```python
from build123d import *

# Parameters (mm, degrees)
REVOLVE_1_ANGLE          = 180
CUT_EXTRUDE_3_DEPTH      = 14.509996299
CUT_EXTRUDE_3_DEPTH_BACK = 14.509996299
SKETCH_5_W               = 6
SKETCH_5_H               = 20
SKETCH_11_R              = 5.65
CUT_EXTRUDE_7_DEPTH      = 13.325988804
SKETCH_12_R              = 6.25
CUT_EXTRUDE_8_DEPTH      = 2


with BuildPart() as part:
    # 草图1 → 旋转1 (revolve)
    with BuildSketch(Plane(origin=(0, 0, 0), x_dir=(0, 0, -1), z_dir=(1, 0, 0))):
        with BuildLine():
            Line((0, 7.8), (0, -7.8))
            ThreePointArc((0, -7.8), (-7.8, 0), (0, 7.8))
        make_face()
    revolve(axis=Axis((0, 7.8, 0), (0, -1, 0)), revolution_arc=REVOLVE_1_ANGLE)

    # 草图5 → 切除-拉伸3 (cut, two sides: drawn at the far end of the back side and taken through both)
    with BuildSketch(Plane.XY.offset(-CUT_EXTRUDE_3_DEPTH_BACK)):
        with Locations((-8.5, 0.096965289)):
            Rectangle(SKETCH_5_W, SKETCH_5_H)
    extrude(amount=CUT_EXTRUDE_3_DEPTH + CUT_EXTRUDE_3_DEPTH_BACK, mode=Mode.SUBTRACT)

    # 草图11 → 切除-拉伸7 (cut, through all)
    with BuildSketch(Plane(origin=(0, 0, 0), x_dir=(0, 0, -1), z_dir=(1, 0, 0))):
        Circle(SKETCH_11_R)
    extrude(amount=-CUT_EXTRUDE_7_DEPTH, mode=Mode.SUBTRACT)

    # 草图12 → 切除-拉伸8 (cut)
    with BuildSketch(Plane(origin=(0, 0, 0), x_dir=(0, 0, -1), z_dir=(1, 0, 0))):
        Circle(SKETCH_12_R)
    extrude(amount=-CUT_EXTRUDE_8_DEPTH, mode=Mode.SUBTRACT)


solid = part.part
```
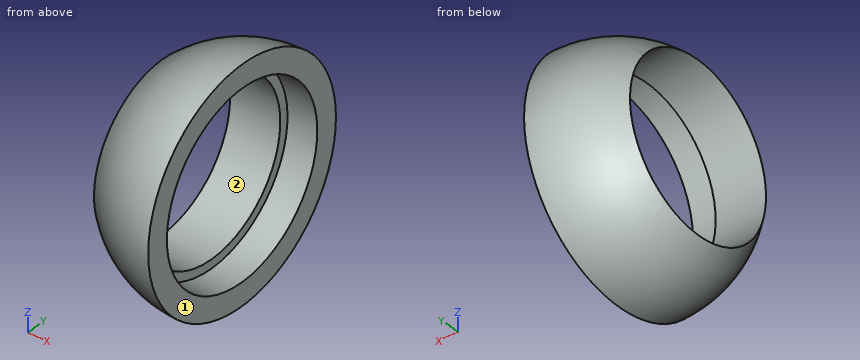
Input: part model. Units: mm. Frame: model coordinates. Face numbers are marked on the shaded views. Round coordinates to 2 decimals unless told otherwise and drop trailing zeros. Loops run counter-clockwise (first coordinate to the right, second up) from the corner with the lowest first, then second, coordinate; pieces in that order, holes last. Notation, with made-up numbers: (-12, -31.5) -> (7, -31.5) arc R31 cw to (7, -0.5) -> close; hole circle Ø11 at (84, -6.5). An arc over 180 degrees is marked (long way). One line per item, written item: value.
(1) Section D-D (z = 6.5). Return the cut outline in (x, y).
Geometry check:
outline: (0, -4.31) -> (0, 4.31) arc R4.31 ccw to start
(2) Pin query (flat end, axial travel): pin 1 (1.5 mm diameter, centred on x = -4, z = -5, fed in from -Y); pin 2 (6 mm diameter, centred on y = 2, z = 0, fed in from +X). Return the tip coordinate at first contact, or that it passes through.
Geometry check:
pin 1: y = -5.37
pin 2: through
(3) Section A-A (z = 0). Return the cut outline in (x, y), plus the area to 3 significant figures.
Geometry check:
outline: (-5.38, -5.65) arc R7.8 ccw to (0, -7.8) -> (0, -6.25) -> (-2, -6.25) -> (-2, -5.65) -> close; (-5.38, 5.65) -> (-2, 5.65) -> (-2, 6.25) -> (0, 6.25) -> (0, 7.8) arc R7.8 ccw to start
area: 13.5 mm2
(4) Mould query, pull axis Z, two halves, no side actions, for the marked faces 1 and 2. Classes: pulls with the +Z half, pulls with the -Z half, needs draft (parallel to the pull), parting line crosses it, or undercut.
Geometry check:
face 1: needs draft
face 2: undercut
(5) Material intervals for line 1 (Y direction, x = -0.85, z = 0); line 2 (Z direction, x = -1.8, y = 2); line 3 (Z direction, x = -3.8, y = 0), sorted ascending. Write a range as [from, to].
Geometry check:
line 1: [-7.75, -6.25], [6.25, 7.75]
line 2: [-7.32, -5.92], [5.92, 7.32]
line 3: [-6.81, -5.65], [5.65, 6.81]
(6) Section C-C (x = -1.4). Return the cut outline in (y, z).
Geometry check:
outline: circle Ø15.35 at (0, 0); hole circle Ø12.5 at (0, 0)
